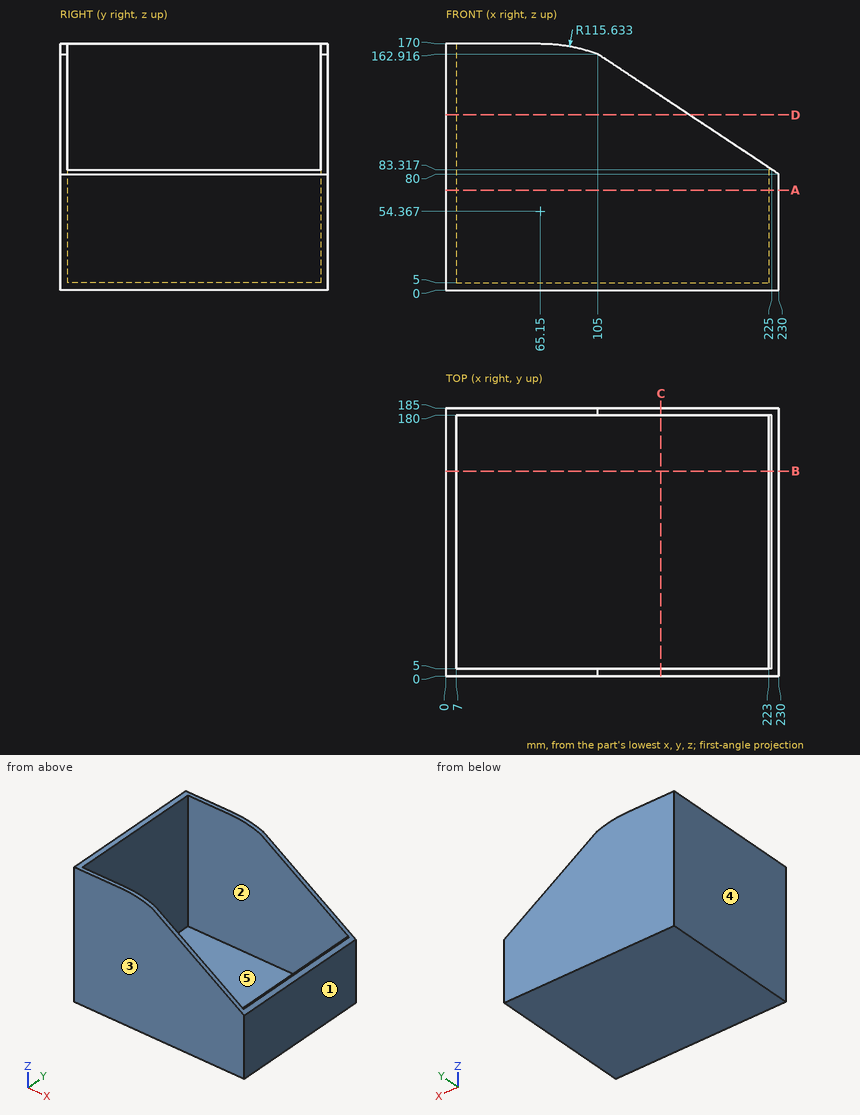
Here's the drawing with two shaded views (mm, measured from the low corner). I have some questions. A direction names the side the tool comes from. Coordinates: 2 decimals unless noted, no trailing zeros. Write each loop counter-clockwise with the first axis right and the second up, starting at its lowest first coordinate (ties: lowest second). Pieces come first, ordered by that corner, then holes. Notation, with made-up numbers: (82.25, 26) -> (97.25, 26) arc R33 ccw to (97.25, 54) -> close; hole circle Ø10 at (-25.5, -13). An arc over 180 degrees is marked (long way). Write item = value, one per line. Start each with the question number.
(1) I want a section at A-A (z = 69). Please give me the cut outline in (x, y).
(2) I need wall thicknesses on line 1 (X direction, y = 64, z = 39); line 2 (Y direction, x = 153.5, z = 49.5); line 3 (X direction, y = 96.5, z = 95). Which ranges of each line are inside material? Lowest first, please. Write a range as [from, to].
(3) I want a section at C-C (x = 148.5). Please give me the cut outline in (y, z).
(4) Which directions (+Z, -Z, +X, -X, +Y, -Y) give clear straight access to the entire face, cutting with the end or side of a thin tool? Please do the marked faces 4 and 5.
(5) Will these pins go through, and if not, where does the flat tip stop? pin 1 (4 mm diameter, centred on x = 93, y = 147, fed in from +Z); pin 2 (1.6 mm diameter, centred on x = 223.5, y = 95.5, fed in from +Z); pin 3 (1.5 mm diameter, centred on y = 54, z = 92.5, fed in from +X).
(6) I want a section at B-B (y = 141.5). Please give me the cut outline in (x, z).
(7) I want a section at D-D (z = 121). Please give me the cut outline in (x, y), plus the area to 3 significant figures.
(8) We'd pull the mould along Y, two halves only. Please class the marked faces 1, 2 and 3: released by +Y, released by -Y, zero draft, split by the parting line, or undercut.
Result set:
q1.outline = (0, 0) -> (230, 0) -> (230, 185) -> (0, 185) -> close; hole (7, 5) -> (223, 5) -> (223, 180) -> (7, 180) -> close
q2.line_1 = [0, 7], [223, 230]
q2.line_2 = [0, 5], [180, 185]
q2.line_3 = [0, 7]
q3.outline = (0, 0) -> (185, 0) -> (185, 134.06) -> (180, 134.06) -> (180, 5) -> (5, 5) -> (5, 134.06) -> (0, 134.06) -> close
q4.face_4 = +Z, -Z, -X, +Y, -Y
q4.face_5 = +Z
q5.pin_1 = 5
q5.pin_2 = 83.32
q5.pin_3 = 7
q6.outline = (0, 0) -> (230, 0) -> (230, 80) -> (225, 83.32) -> (223, 83.32) -> (223, 5) -> (7, 5) -> (7, 170) -> (0, 170) -> close
q7.outline = (0, 0) -> (168.19, 0) -> (168.19, 5) -> (7, 5) -> (7, 180) -> (168.19, 180) -> (168.19, 185) -> (0, 185) -> close
q7.area = 2,910 mm2
q8.face_1 = zero draft
q8.face_2 = undercut
q8.face_3 = released by -Y
